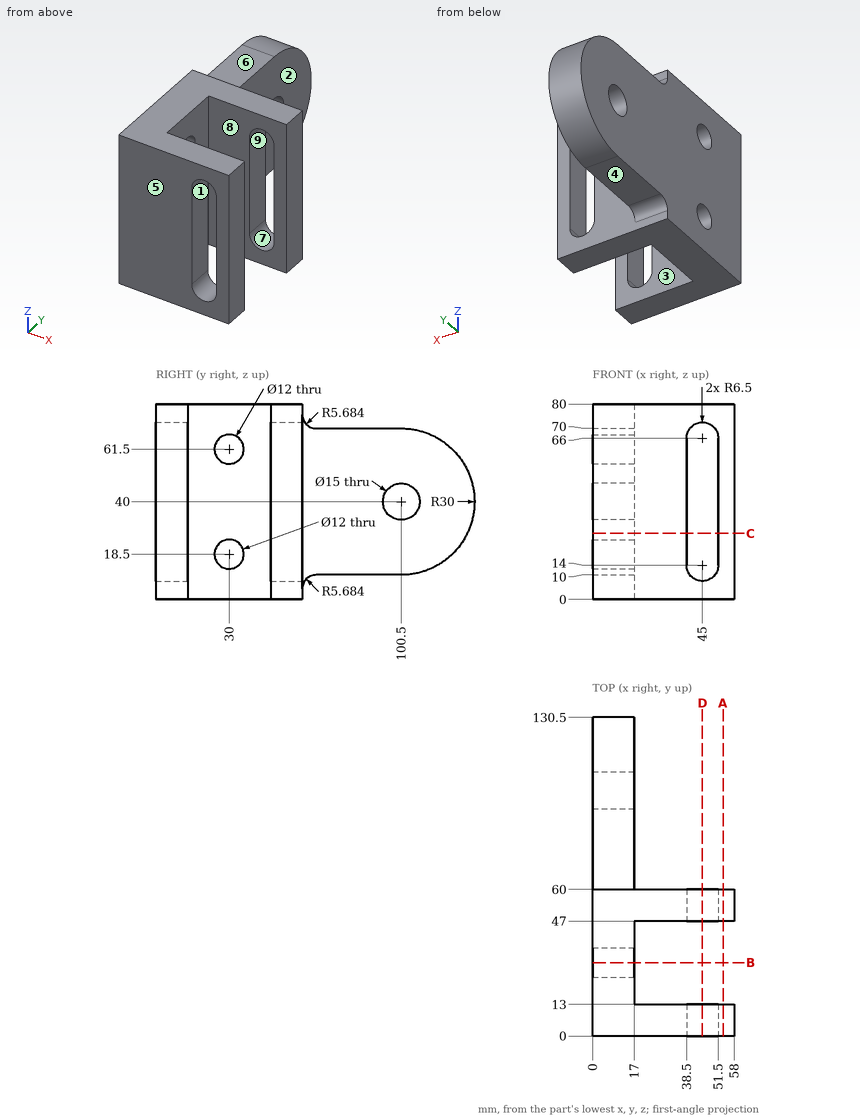
Design review of the part shown in the three views and the two pictorial views. Dimensions are in mm from the part's minimum x, y and z. A direction names the side the tool comes from. Coordinates: 2 decimals unless noted, no trailing zeros. Order: outer loops, then holes, each group sorted by start corner. A loop starts at its lowest first (then second) coordinate and runs counter-clockwise, first axis right, second up.
Item 1: Take a section at C-C, the plane z = 27. Write out the cut boundary in (x, y).
Item 2: The part is to be moulded in two halves that separate along Z. For the marked faces 6, 7, 8 and 9, say which applies: pulls with the +Z half, pulls with the -Z half, needs draft (parallel to the pull), parting line crosses it, or undercut.
Item 3: Take a section at A-A, the plane x = 53.5. Write out the cut boundary in (y, z).
Item 4: For pin 1 Ø10 at (y, z) = (23, 20) entering from +X; pin 2 Ø8.5 at (x, y) = (8, 77.5) entering from +Z; pin 3 Ø12.5 at (x, z) = (33, 50) entering from +Y, all flat-tipped, find the tip position at first contact; note any pin that passes through.
Item 5: Take a section at D-D, the plane x = 45. Write out the cut boundary in (y, z).
Item 6: For line 1 (Z direction, x = 7.5, y = 30); line 2 (Y direction, x = 19, z = 33.5); line 3 (Z direction, x = 12.5, y = 100.5), list the stretches that pass through material, from the lowest coordinate up.
Item 7: Take a section at B-B, the plane y = 30. Write out the cut boundary in (x, z), then the cut area to 3 significant figures.
Item 8: For the marked faces 1, 2, 3, 4 and 5, list the 3-axis set-ups (+Z, -Z, +X, -X, +Y, -Y) from which the entire face can be reached by the end or side of a thin tool; tool diameter is ignored.
The answers:
1. outline: (0, 0) - (38.5, 0) - (38.5, 13) - (17, 13) - (17, 47) - (38.5, 47) - (38.5, 60) - (17, 60) - (17, 127.54) - (0, 127.54) - close; (51.5, 0) - (58, 0) - (58, 13) - (51.5, 13) - close; (51.5, 47) - (58, 47) - (58, 60) - (51.5, 60) - close
2. face 6: pulls with the +Z half
2. face 7: undercut
2. face 8: needs draft
2. face 9: undercut
3. outline: (0, 0) - (13, 0) - (13, 80) - (0, 80) - close; (47, 0) - (60, 0) - (60, 80) - (47, 80) - close
4. pin 1: stops at x = 17
4. pin 2: stops at z = 70
4. pin 3: stops at y = 60
5. outline: (0, 0) - (13, 0) - (13, 7.5) - (0, 7.5) - close; (0, 72.5) - (13, 72.5) - (13, 80) - (0, 80) - close; (47, 0) - (60, 0) - (60, 7.5) - (47, 7.5) - close; (47, 72.5) - (60, 72.5) - (60, 80) - (47, 80) - close
6. line 1: z = 0 to 12.5, 24.5 to 55.5, 67.5 to 80
6. line 2: y = 0 to 13, 47 to 60
6. line 3: z = 10 to 32.5, 47.5 to 70
7. outline: (0, 0) - (17, 0) - (17, 12.5) - (0, 12.5) - close; (0, 24.5) - (17, 24.5) - (17, 55.5) - (0, 55.5) - close; (0, 67.5) - (17, 67.5) - (17, 80) - (0, 80) - close
7. area: 952 mm2
8. face 1: +Y, -Y
8. face 2: +Z, -Z, +X, +Y
8. face 3: +Z, -Z, +X
8. face 4: -Z, +X, -X, +Y
8. face 5: +Z, -Z, +X, -X, -Y
